The listing builds one solid part. Answer for the finished solid, in the listing's coordinates (mm). A direction names the side the tool comes from. Give positions to 0.01 mm unless a question says otherwise; leave off trailing zeros. Order: outer loops, then holes, each group sorted by start corner. A loop starts at its lowest first (then second) coordinate and runs counter-clockwise, first axis right, second up. Notation, with made-up numbers: (22.25, 70.5) - (76.25, 70.5) arc R17 ccw to (76.25, 102.5) - close; hole circle Ø9 at (-33, 44.25). An arc over 180 degrees is marked (long way). Answer as a JSON object with one key per item and string values. Group by question number.
Q1. A cutting plane is placed at A-A, the plane y = 147. Give the vertices of the cut face in (x, z).
Q2. The mould has two halves that part along X. Classify faces 3 (the face through (0, 617, 12.7)), 4 (the face through (-23, 602, 0)), 5 (the face through (0, 617, -12.65)), 6 (the face through (-1, 1221, 23.876)): released by +X, released by -X, zero draft, split by the parting line, or undercut.
Q3. A cutting plane is placed at B-B, the plane z = 1. Give the vertices of the cut face in (x, y), and give its area (3 significant figures).
Q4. Consider line 1 (Y direction, x = -4, z = -14.5); line 2 (X direction, y = 577, z = 14); line 3 (Y direction, x = 1.5, z = -21). Determine where each line is inside the solid, lowest interval first.
Q5. Given pin 1 (2 mm diameter, centred on y = 566, z = -1, fed in from +X); pin 2 (6 mm diameter, centred on x = 2.5, y = 768.5, fed in from -Z); pin 3 (14 mm diameter, centred on x = -2, y = 796, fed in from +Z), each flat-ended and moving along its own axis, determine where each tip first touches the part or whether it passes through.
Q6. For faces 1 (the face through (23, 618, 0)), 2 (the face through (-1, 1, 23.876)), determine the directions among +Z, -Z, +X, -X, +Y, -Y from which every point of the face is accessible in a straight line to the end or side of a thin tool.
from build123d import *

# Parameters (mm, degrees)
EXTRUDE1_DEPTH      = 19.05
EXTRUDE1_DEPTH_BACK = 19
CUT_EXTRUDE1_DEPTH  = 6.35
CUT_EXTRUDE2_DEPTH  = 6.35
SKETCH6_R           = 47.657715
SKETCH6_R_2         = 47.657166
EXTRUDE2_DEPTH      = 4.826
EXTRUDE2_DEPTH_BACK = 43.18


with BuildPart() as part:
    # Sketch3 → Extrude1 (new body, two sides)
    with BuildSketch(Plane.XY) as extrude1_sk:
        with BuildLine():
            Line((23, 1178.259012), (23, 41.73971))
            ThreePointArc((23, 41.73971), (0, -47.657144), (-23, 41.73971))
            Line((-23, 41.73971), (-23, 1178.259012))
            ThreePointArc((-23, 1178.259012), (0, 1267.657089), (23, 1178.259012))
        make_face()
    extrude(amount=EXTRUDE1_DEPTH)
    extrude(extrude1_sk.sketch, amount=-EXTRUDE1_DEPTH_BACK)

    # Sketch4 → Cut-Extrude1 (cut)
    with BuildSketch(Plane.XY.offset(19.05)):
        with BuildLine():
            Line((15.888, 1116.347374), (15.888, 103.651374))
            ThreePointArc((15.888, 103.651374), (13.060995, 96.826379), (6.236, 93.999374))
            Line((6.236, 93.999374), (-6.236, 93.999374))
            ThreePointArc((-6.236, 93.999374), (-13.060995, 96.826379), (-15.888, 103.651374))
            Line((-15.888, 103.651374), (-15.888, 1116.347374))
            ThreePointArc((-15.888, 1116.347374), (-13.060995, 1123.172368), (-6.236, 1125.999374))
            Line((-6.236, 1125.999374), (6.236, 1125.999374))
            ThreePointArc((6.236, 1125.999374), (13.060995, 1123.172368), (15.888, 1116.347374))
        make_face()
    extrude(amount=-CUT_EXTRUDE1_DEPTH, mode=Mode.SUBTRACT)

    # Sketch5 → Cut-Extrude2 (cut)
    with BuildSketch(Plane(origin=(0, 0, -19), x_dir=(-1, 0, 0), z_dir=(0, 0, -1))):
        with BuildLine():
            Line((-15.888, 1116.347374), (-15.888, 103.651374))
            ThreePointArc((-15.888, 103.651374), (-13.060995, 96.826379), (-6.236, 93.999374))
            Line((-6.236, 93.999374), (6.236, 93.999374))
            ThreePointArc((6.236, 93.999374), (13.060995, 96.826379), (15.888, 103.651374))
            Line((15.888, 103.651374), (15.888, 1116.347374))
            ThreePointArc((15.888, 1116.347374), (13.060995, 1123.172368), (6.236, 1125.999374))
            Line((6.236, 1125.999374), (-6.236, 1125.999374))
            ThreePointArc((-6.236, 1125.999374), (-13.060995, 1123.172368), (-15.888, 1116.347374))
        make_face()
    extrude(amount=-CUT_EXTRUDE2_DEPTH, mode=Mode.SUBTRACT)

    # Sketch6 → Extrude2 (add, two sides)
    with BuildSketch(Plane.XY.offset(19.05)) as extrude2_sk:
        with Locations((0, 1219.999374)):
            Circle(SKETCH6_R)
        Circle(SKETCH6_R_2)
    extrude(amount=EXTRUDE2_DEPTH)
    extrude(extrude2_sk.sketch, amount=-EXTRUDE2_DEPTH_BACK)


solid = part.part
Reply:
{
 "1": {"outline": "(-23, -19) - (-15.89, -19) - (-15.89, -12.65) - (15.89, -12.65) - (15.89, -19) - (23, -19) - (23, 19.05) - (15.89, 19.05) - (15.89, 12.7) - (-15.89, 12.7) - (-15.89, 19.05) - (-23, 19.05) - close"},
 "2": {"face 3": "undercut", "face 4": "released by -X", "face 5": "undercut", "face 6": "zero draft"},
 "3": {"outline": "(-23, 41.74) arc R47.66 ccw (long way) to (23, 41.74) - (23, 1178.26) arc R47.66 ccw (long way) to (-23, 1178.26) - close", "area": "66,200 mm^2"},
 "4": {"line 1": "y = -47.49 to 94, 1126 to 1267.49", "line 2": "x = -23 to -15.89, 15.89 to 23", "line 3": "y = -47.63 to 47.63, 1172.37 to 1267.63"},
 "5": {"pin 1": "stops at x = 23", "pin 2": "stops at z = -12.65", "pin 3": "stops at z = 12.7"},
 "6": {"face 1": "+Z, -Z, +X", "face 2": "+Z, +X, -X, +Y, -Y"}
}
